from build123d import *

# Parameters (mm, degrees)
ESQUISSE1_W             = 30
ESQUISSE1_H             = 12
BOSS_EXTRU_1_DEPTH      = 2
ESQUISSE2_R             = 3.25
BOSS_EXTRU_2_DEPTH      = 0.5
ESQUISSE3_R             = 2.4
BOSS_EXTRU_3_DEPTH      = 4.2
ESQUISSE6_W             = 6.7
ESQUISSE6_H             = 17
BOSS_EXTRU_4_DEPTH      = 4.2
ESQUISSE8_W             = 4.2
ESQUISSE8_H             = 5
BOSS_EXTRU_5_DEPTH      = 2
CONG_1_R                = 3
BOSS_EXTRU_6_START      = -4.2
BOSS_EXTRU_6_DEPTH      = 4.2
ESQUISSE12_W            = 4.2
ESQUISSE12_H            = 12.517587627
BOSS_EXTRU_8_DEPTH      = 65
ESQUISSE13_R            = 2.5
ENL_V_MAT_EXTRU_2_DEPTH = 4.2


with BuildPart() as part:
    # Esquisse1 → Boss.-Extru.1 (new body)
    with BuildSketch(Plane.XY):
        with Locations((2.190701098, -1.023529412)):
            Rectangle(ESQUISSE1_W, ESQUISSE1_H)
    extrude(amount=BOSS_EXTRU_1_DEPTH)

    # Esquisse2 → Boss.-Extru.2 (add)
    with BuildSketch(Plane.XY.offset(2)):
        with Locations((8.190701098, -1.023529412)):
            Circle(ESQUISSE2_R)
        with Locations((-3.809298902, -1.023529412)):
            Circle(ESQUISSE2_R)
    extrude(amount=BOSS_EXTRU_2_DEPTH)

    # Esquisse3 → Boss.-Extru.3 (add)
    with BuildSketch(Plane.XY.offset(2.5)):
        with Locations((-3.809298902, -1.023529412)):
            Circle(ESQUISSE3_R)
        with Locations((8.190701098, -1.023529412)):
            Circle(ESQUISSE3_R)
    extrude(amount=BOSS_EXTRU_3_DEPTH)

    # Esquisse6 → Boss.-Extru.4 (add)
    with BuildSketch(Plane(origin=(17.190701098, 0, 0), x_dir=(0, 0, -1), z_dir=(1, 0, 0))):
        with Locations((-3.35, -3.523529412)):
            Rectangle(ESQUISSE6_W, ESQUISSE6_H)
    extrude(amount=BOSS_EXTRU_4_DEPTH)

    # Esquisse8 → Boss.-Extru.5 (add)
    with BuildSketch(Plane.XY.offset(6.7)):
        with Locations((19.290701098, -9.523529412)):
            Rectangle(ESQUISSE8_W, ESQUISSE8_H)
    extrude(amount=BOSS_EXTRU_5_DEPTH)

    # Congé1
    cong_1_edges = [part.edges().sort_by_distance(p)[0] for p in [
        (21.390701098, 4.976470588, 3.35),
        (-12.809298902, 4.976470588, 1),
        (-12.809298902, -7.023529412, 1),
    ]]
    fillet(cong_1_edges, radius=CONG_1_R)

    # Esquisse9 → Boss.-Extru.6 (add)
    with BuildSketch(Plane(origin=(21.390701098, 0, 0), x_dir=(0, 0, -1), z_dir=(1, 0, 0)).offset(BOSS_EXTRU_6_START)):
        Polygon((-8.7, -12.023529412), (-8.7, -21.023529412), (0, -12.023529412), align=None)
    extrude(amount=BOSS_EXTRU_6_DEPTH)

    # Esquisse12 → Boss.-Extru.8 (add)
    with BuildSketch(Plane(origin=(0, -5.808034598, -6.008311653), x_dir=(1, 0, 0), z_dir=(0, -0.6950220968474751, -0.7189883760491119))):
        with Locations((19.290701098, 14.9035717)):
            Rectangle(ESQUISSE12_W, ESQUISSE12_H)
    extrude(amount=BOSS_EXTRU_8_DEPTH)

    # Esquisse13 → Enlèv. mat.-Extru.2 (cut)
    with BuildSketch(Plane.ZY.offset(-17.190701098)):
        with Locations(Location((-35.913349059, -55.444766835, 0), (0, 0, 270))):
            Circle(ESQUISSE13_R)
    extrude(amount=-ENL_V_MAT_EXTRU_2_DEPTH, mode=Mode.SUBTRACT)


solid = part.part
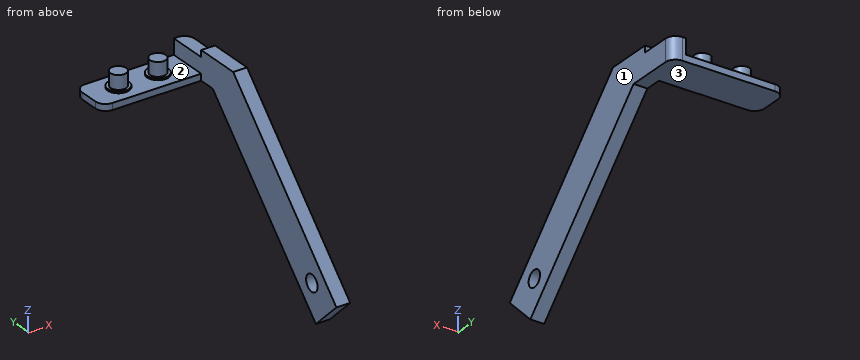
Read the model definition and answer for the solid it produces. Units are mm, in the model's axes. Face numbers are marked on the shaded views. A direction names the side the tool comes from. Round coordinates to 2 decimals unless told otherwise and drop trailing zeros. Write each loop counter-clockwise with the first axis right and the second up, starting at its lowest first coordinate (ties: lowest second). Pieces come first, ordered by that corner, then holes.
Q1. A tool of negligible diameter and unlimited length cuts with its end or side. For the marked faces 1, 2 and 3, from which of +Z, -Z, +X, -X, +Y, -Y can it reach the whole face along a straight path? Write none if from no direction.
Values:
face 1: +Z, -Z, +X, +Y, -Y
face 2: +Z
face 3: -Z, +X, -X, +Y
Q2. Straight lines are drawn through the part: line 1 (X direction, y = -33, z = -17.5); line 2 (Y direction, x = 8, z = 5); line 3 (Z direction, x = -3, y = -2.5). For each, find the intervals that lie inside material, in ascending order.
Values:
line 1: x = 17.19 to 21.39
line 2: y = -3.42 to 1.37
line 3: z = 0 to 6.7
Q3. Find section A-A on z = 5. Determine the outline of the cut face in (x, y).
Values:
outline: circle Ø4.8 at (-3.81, -1.02); circle Ø4.8 at (8.19, -1.02); (17.19, -24.6) - (21.39, -24.6) - (21.39, 1.98) arc R3 ccw to (18.39, 4.98) - (17.19, 4.98) - close
Q4. Flat-ended cylindrical pins translate along their axes: P1, Ø1.4, axis at x = 7, y = 0, coming from the +Z side; P2, Ø1, axis at x = 3.5, z = 1, coming from the -Y side; P3, Ø18.5, axis at x = 3.5, y = -4.5, coming from the -Z side. Find the tip coordinate at first contact, or state that the pin passes through.
Values:
P1: stops at z = 6.7
P2: stops at y = -7.02
P3: stops at z = 0
Q5. Find section B-B on y = -2.5. Determine the outline of the cut face in (x, z), and give its area (3 significant figures).
Values:
outline: (-12.81, 0) - (21.39, 0) - (21.39, 6.7) - (17.19, 6.7) - (17.19, 2) - (11.09, 2) - (11.09, 2.5) - (10.08, 2.5) - (10.08, 6.7) - (6.3, 6.7) - (6.3, 2.5) - (5.3, 2.5) - (5.3, 2) - (-0.91, 2) - (-0.91, 2.5) - (-1.92, 2.5) - (-1.92, 6.7) - (-5.7, 6.7) - (-5.7, 2.5) - (-6.7, 2.5) - (-6.7, 2) - (-12.81, 2) - close
area: 126 mm2
Q6. Find section C-C on x = 1.5. Determine the outline of the cut face in (y, z).
Values:
outline: (-7.02, 0) - (4.98, 0) - (4.98, 2) - (-7.02, 2) - close
Q7. Find section D-D on z = -1.5. Determine the outline of the cut face in (x, y).
Values:
outline: (17.19, -30.88) - (21.39, -30.88) - (21.39, -13.47) - (17.19, -13.47) - close
